Work out the finished part from the listing and answer in its coordinate system (mm). Face numbers are marked on the shaded views. A direction names the side the tool comes from. Round coordinates to 2 decimals unless told otherwise and drop trailing zeros. Loops run counter-clockwise (first coordinate to the right, second up) from the corner with the lowest first, then second, coordinate; pieces in that order, holes last. Notation, with made-up numbers: M 14.5,-10.75 L 66.5,-10.75 A6 ccw 66.5,-4.75 Z; hole C 25,85.5 d11. An arc over 180 degrees is marked long. One line per item, written item: value.
Autodesk Inventor part; units mm, degrees
ref_plane "YZ Plane" through (0, 0, 0) normal (1, 0, 0) x (0, 1, 0)
ref_plane "XZ Plane" through (0, 0, 0) normal (0, 1, 0) x (-1, 0, 0)
ref_plane "XY Plane" through (0, 0, 0) normal (0, 0, 1) x (1, 0, 0)
sketch "Sketch1" plane through (0, 0, 0) normal (0, 0, 1) x (1, 0, 0)
  line L0 (33, -19) -> (-33, -19)
  line L1 (-33, -19) -> (-33, 19)
  line L2 (-33, 19) -> (33, 19)
  line L3 (33, 19) -> (33, -19)
  line L4 (33, -19) -> (-33, 19) construction
  line L5 (-33, -19) -> (33, 19) construction
  point P0 (0, 0)
  dimension "d0" = 66
  dimension "d1" = 38
extrude "Extrusion1" add sketch "Sketch1" along normal blind 9.5
sketch "Sketch2" plane through (0, 0, 0) normal (0, 0, -1) x (-1, 0, 0)
  line L0 (-31, -7) -> (31, -7)
  line L1 (31, -7) -> (31, -17)
  line L2 (31, -17) -> (-31, -17)
  line L3 (-31, -17) -> (-31, -7)
  line L4 (33, 19) -> (33, -19)
  line L5 (-33, -19) -> (-33, 19) construction
  line L6 (33, 19) -> (33, -19) construction
  line L7 (33, -19) -> (-33, -19) construction
  point P0 (0, 0)
  point P1 (0, -7)
  dimension "d4" = 2
  dimension "d5" = 2
  dimension "d6" = 12
extrude "Extrusion2" cut sketch "Sketch2" against normal blind 7
sketch "Sketch3" plane through (0, 0, 9.5) normal (0, 0, 1) x (1, 0, 0)
  line L0 (33, -19) -> (33, 19)
  line L1 (-33, 19) -> (33, 19) construction
  line L2 (33, 19) -> (33, 8) construction
  line L3 (33, 8) -> (-33, 8) construction
  line L4 (-33, 8) -> (-33, 19) construction
  line L5 (-33, -19) -> (33, -19)
  line L6 (-33, 8) -> (33, 8)
  line L7 (33, 8) -> (33, 12.5)
  line L8 (33, 12.5) -> (-33, 12.5)
  line L9 (-33, 12.5) -> (-33, 8)
  line L10 (33, 19) -> (-33, 19)
  line L11 (-33, 19) -> (33, 19)
  line L12 (33, 19) -> (33, 14.5)
  line L13 (33, 14.5) -> (-33, 14.5)
  line L14 (-33, 14.5) -> (-33, 19)
  point P0 (0, 0)
  dimension "d9" = 27
  dimension "d10" = 2
  dimension "d11" = 4.5
extrude "Extrusion3" add sketch "Sketch3" along normal blind 15
sketch "Sketch4" plane through (0, 0, 9.5) normal (0, 0, 1) x (1, 0, 0)
  line L0 (-33, 14.5) -> (-33, 12.5)
  line L1 (-33, 12.5) -> (33, 12.5)
  line L2 (-33, 14.5) -> (33, 14.5)
  line L3 (33, 14.5) -> (33, 12.5)
  line L4 (33, 12.5) -> (-33, 12.5)
  line L5 (-33, 12.5) -> (-33, 14.5)
  point P0 (0, 0)
extrude "Extrusion4" add sketch "Sketch4" along normal blind 3
chamfer "Chamfer1" distance 2 angle 45 8 edges at (33, 12.5, 18.5) (33, 8, 17) (-33, 12.5, 18.5) (-33, 8, 17) (-33, 19, 12.25) (-33, 14.5, 18.5) (33, 14.5, 18.5) (33, 19, 12.25)
sketch "Sketch5" plane through (0, 0, 9.5) normal (0, 0, 1) x (1, 0, 0)
  circle A0 centre (-22.1, 0.05) radius 5.5
  circle A1 centre (21.9, 0.05) radius 5.5
  line L0 (33, -19) -> (33, 10)
  line L1 (-33, -19) -> (33, -19)
  point P0 (0, 0)
  dimension "d19" = 11
  dimension "d20" = 11
  dimension "d21" = 44
  dimension "d22" = 11.1
  dimension "d23" = 19.05
hole "Hole1" at (-22.1, 0.05, 9.5) at (21.9, 0.05, 9.5) direction (0, 0, -1) diameter 5.5 end through all counterbore diameter 8.5 counterbore depth 5
equation "\"d11\" = -0.5 * d10 + 0.5 * d1 - 0.5 * d9"
equation "\"d20\" = d19"
properties part number "Floor_support_dammy"
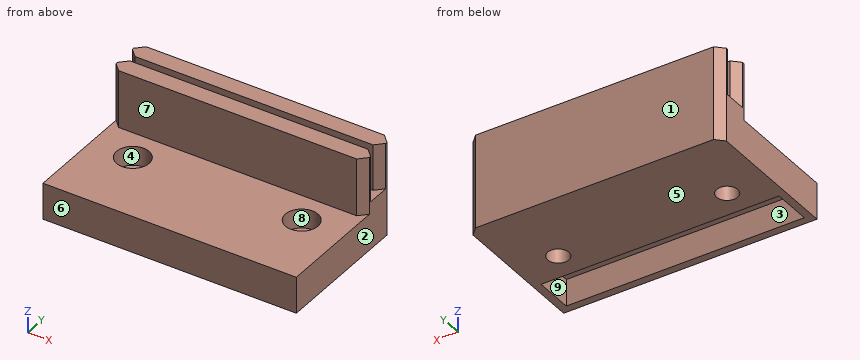
1) For the marked faces 5, 6, 7, 8 and 9, determine the directions among +Z, -Z, +X, -X, +Y, -Y from which every point of the face is accessible in a straight line to the end or side of a thin tool.
Check values:
face 5: -Z, +X, -X, +Y, -Y
face 6: +Z, -Z, +X, -X, -Y
face 7: +Z, +X, -X, -Y
face 8: +Z
face 9: -Z
2) Find section A-A (z = 17.25). Give the vertices of the cut face in (x, y).
Check values:
outline: M -33,10 L -31,8 L 31,8 L 33,10 L 33,10.5 L 31,12.5 L -31,12.5 L -33,10.5 Z; M -33,16.5 L -31,14.5 L 31,14.5 L 33,16.5 L 33,17 L 31,19 L -31,19 L -33,17 Z
3) The mould has two halves that part along X. Classify the marked faces 1, 2, 3 and 4: +X half, -X half, draft (parallel to the pull), parting line (faces both ways), or undercut.
Check values:
face 1: draft
face 2: +X half
face 3: undercut
face 4: undercut
4) Find section B-B (x = 21.9). Give the vertices of the cut face in (y, z).
Check values:
outline: M -19,0 L -17,0 L -17,7 L -7,7 L -7,0 L -2.7,0 L -2.7,4.5 L -4.2,4.5 L -4.2,9.5 L -19,9.5 Z; M 2.8,0 L 19,0 L 19,24.5 L 14.5,24.5 L 14.5,12.5 L 12.5,12.5 L 12.5,24.5 L 8,24.5 L 8,9.5 L 4.3,9.5 L 4.3,4.5 L 2.8,4.5 Z
5) Each of these flat-tipped pins is pushed along its axis until it touches: pin 1 (10 mm diameter, centred on x = 5, y = -12, fed in from +Z); pin 2 (5 mm diameter, centred on x = -5, z = 14, fed in from -Y); pin 3 (7 mm diameter, centred on x = -22.1, y = 0.05, fed in from +Z). Where does it stop, or does it pass through?
Check values:
pin 1: z = 9.5
pin 2: y = 8
pin 3: z = 4.5
6) Find section D-D (z = 3.75). Give the vertices of the cut face in (x, y).
Check values:
outline: M -33,-19 L 33,-19 L 33,17 L 31,19 L -31,19 L -33,17 Z; hole M -31,-17 L 31,-17 L 31,-7 L -31,-7 Z; hole C -22.1,0.05 d5.5; hole C 21.9,0.05 d5.5
7) Find the intervals of material crossed by probe 1 along Y at (x, z) = (-22.1, 2.2); probe 2 along X at (y, z) = (0.05, 7.8); probe 3 along X at (y, z) = (0.05, 2.4), in increasing order. Write a range as from..to.
Check values:
probe 1: -19..-17, -7..-2.7, 2.8..19
probe 2: -33..-26.35, -17.85..17.65, 26.15..33
probe 3: -33..-24.85, -19.35..19.15, 24.65..33
8) Find section C-C (y = 0.05). Give the vertices of the cut face in (x, z).
Check values:
outline: M -33,0 L -24.85,0 L -24.85,4.5 L -26.35,4.5 L -26.35,9.5 L -33,9.5 Z; M -19.35,0 L 19.15,0 L 19.15,4.5 L 17.65,4.5 L 17.65,9.5 L -17.85,9.5 L -17.85,4.5 L -19.35,4.5 Z; M 24.65,0 L 33,0 L 33,9.5 L 26.15,9.5 L 26.15,4.5 L 24.65,4.5 Z
